For this review, take the finished solid that the model builds, in its own axes (mm). A direction names the side the tool comes from. Coordinates: 2 decimals unless noted, no trailing zeros. Order: outer loops, then holes, each group sorted by start corner. A loop starts at its lowest first (then second) coordinate and runs counter-clockwise, first axis right, second up. Notation, with made-up numbers: (37.5, 86) - (56.5, 86) arc R30 cw to (56.5, 123) - close; hole circle Ø8 at (89.5, 12). An arc over 180 degrees is marked (long way). One line per item, written item: value. Start each with the question number.
(1) Consider section A-A on z = 5. Write out the cut boundary in (x, y), then the cut area to 3 significant figures.
(2) Consider section D-D on y = 10. Write out the cut boundary in (x, z).
(3) Clearance check with flat-ended pins moving along their axes: pin 1 (0.7 mm diameter, centred on x = -0.5, z = 2, fed in from +Y); pin 2 (0.7 mm diameter, centred on x = 5.5, y = 2.5, fed in from -Z); pin 3 (5 mm diameter, centred on x = 2.54, y = 15.77, fed in from +Z). State where each tip first meets the part, or that it passes through.
(4) Mouldability with a two-part tool opening along Y and no side actions: class faces 1 (the flat face through (2.47, 12.15, -1.73)), 2 (the flat face through (2.5, 1, -1.28)), 3 (the flat face through (5.96, 0, 1)) as released by +Y, released by -Y, zero draft, split by the parting line, or undercut.
(5) Consider section B-B on x = 2.54. Write out the cut boundary in (y, z) (3 decimals).
(6) Consider section C-C on y = 15.77. Write out the cut boundary in (x, z) (3 decimals).
(7) To check wall thickness, follow line 1 along Y through (x, z) = (2.54, -4.35) (3 decimals); line 2 along Z through (x, y) = (6.5, 17); line 3 along Z through (x, y) = (5, 10.5). State the ranges of each line that lie inside material, in increasing order.
(8) For faces 4 (the cylindrical face through (2.5, -2.2, -1.1)), 5 (the flat face through (-0.88, 0, 1)), 6 (the flat face through (2.5, 1, -1.92)), 7 (the flat face through (3, 7, 0)), list the 3-axis set-ups (+Z, -Z, +X, -X, +Y, -Y) from which the entire face can be reached by the end or side of a thin tool; tool diameter is ignored.
```python
from build123d import *

# Parameters (mm, degrees)
SKETCH_5_W                      = 10.3
SKETCH_5_H                      = 4.8
EXTRUDE_1_DEPTH                 = 15.75
CUT_EXTRUDE_1_REACH             = 23.278
CUT_EXTRUDE_1_DIRECTION_2_REACH = 23.278
SKETCH_11_R                     = 1.865
CUT_EXTRUDE_2_DEPTH             = 4.8
SKETCH_3_W                      = 0.84
SKETCH_3_H                      = 0.64
SKETCH_4_W                      = 0.84
SKETCH_4_H                      = 0.64
SKETCH_3_3_W                    = 0.84
SKETCH_3_3_H                    = 0.64
EXTRUDE_2_DEPTH                 = 2.5
SKETCH_4_3_W                    = 0.84
SKETCH_4_3_H                    = 0.64
EXTRUDE_3_DEPTH                 = 2.5
SKETCH_12_W                     = 0.84
SKETCH_12_H                     = 0.64
EXTRUDE_4_DEPTH                 = 4
EXTRUDE_5_DEPTH                 = 0.46
EXTRUDE_6_DEPTH                 = 0.46
CUT_EXTRUDE_3_DEPTH             = 0.46
CUT_EXTRUDE_START               = -0.46
CUT_EXTRUDE_4_DEPTH             = 0.46
SKETCH_17_R                     = 0.172950306
CUT_EXTRUDE_5_DEPTH             = 2
SKETCH_18_W                     = 11.930877945
SKETCH_18_H                     = 3.370946467
CUT_EXTRUDE_6_DEPTH             = 2
EXTRUDE_7_DEPTH                 = 0.84


with BuildPart() as part:
    # Эскиз5 → Вытянуть1 (new body)
    with BuildSketch(Plane(origin=(0, 3.5, 0), x_dir=(-1, 0, 0), z_dir=(0, 1, 0))):
        with Locations((-2.54, -2.4)):
            Rectangle(SKETCH_5_W, SKETCH_5_H)
    extrude(amount=EXTRUDE_1_DEPTH)

    # Вырез-Вытянуть1: up to this face of the body (flat: up to its plane)
    cut_extrude_1_end = Plane(part.part.faces().sort_by_distance((-2.61, 11.375, -2.4))[0])
    # Эскиз10 → Вырез-Вытянуть1 (cut, up to the picked face)
    with BuildSketch(Plane(origin=(0, 0, 0), x_dir=(0, 0, -1), z_dir=(1, 0, 0)), mode=Mode.PRIVATE) as cut_extrude_1_sk1:
        Polygon((0, 19.25), (3.41, 19.25), (3.41, 12.78), (0, 11.5), align=None)
    cut_extrude_1_tool1 = split(extrude(cut_extrude_1_sk1.sketch, amount=-CUT_EXTRUDE_1_REACH, mode=Mode.PRIVATE), bisect_by=cut_extrude_1_end, keep=Keep.BOTH, mode=Mode.PRIVATE)
    add(cut_extrude_1_tool1.solids().sort_by(Axis((0, 15.685398, -1.653842), (-1, 0, 0)))[0], mode=Mode.SUBTRACT)

    # Вырез-Вытянуть1 direction 2: up to this face of the body (flat: up to its plane)
    cut_extrude_1_direction_2_end = Plane(part.part.faces().sort_by_distance((7.69, 11.375, -2.4))[0])
    # Эскиз10 → Вырез-Вытянуть1 direction 2 (cut, up to the picked face)
    with BuildSketch(Plane(origin=(0, 0, 0), x_dir=(0, 0, -1), z_dir=(1, 0, 0)), mode=Mode.PRIVATE) as cut_extrude_1_direction_2_sk1:
        Polygon((0, 19.25), (3.41, 19.25), (3.41, 12.78), (0, 11.5), align=None)
    cut_extrude_1_direction_2_tool1 = split(extrude(cut_extrude_1_direction_2_sk1.sketch, amount=CUT_EXTRUDE_1_DIRECTION_2_REACH, mode=Mode.PRIVATE), bisect_by=cut_extrude_1_direction_2_end, keep=Keep.BOTH, mode=Mode.PRIVATE)
    add(cut_extrude_1_direction_2_tool1.solids().sort_by(Axis((0, 15.685398, -1.653842), (1, 0, 0)))[0], mode=Mode.SUBTRACT)

    # Эскиз11 → Вырез-Вытянуть2 (cut)
    with BuildSketch(Plane.XY):
        with Locations((2.54, 15.77)):
            Circle(SKETCH_11_R)
    extrude(amount=-CUT_EXTRUDE_2_DEPTH, mode=Mode.SUBTRACT)

    # По траектории1: sweep along a path in Эскиз8
    with BuildLine(Plane(origin=(0, 0, 0), x_dir=(0, 0, -1), z_dir=(1, 0, 0))) as sweep_1_path:
        Line((0, 0), (0.6, 0))
        ThreePointArc((0.6, 0), (1.307106781, 0.292893219), (1.6, 1))
        Line((1.6, 1), (1.6, 3.5))
    # Эскиз3 → По траектории1 (sweep)
    with BuildSketch(Plane.XY):
        Rectangle(SKETCH_3_W, SKETCH_3_H)
        with Locations((5.08, 0)):
            Rectangle(SKETCH_3_W, SKETCH_3_H)
    sweep(path=sweep_1_path.line)

    # По траектории2: sweep along a path in Эскиз9
    with BuildLine(Plane(origin=(0, 0, 0), x_dir=(0, 0, -1), z_dir=(1, 0, 0))) as sweep_2_path:
        Line((0, -2.54), (0.6, -2.54))
        ThreePointArc((0.6, -2.54), (1.307106781, -2.247106781), (1.6, -1.54))
        Line((1.6, -1.54), (1.6, 4.77))
    # Эскиз4 → По траектории2 (sweep)
    with BuildSketch(Plane.XY):
        with Locations((2.54, -2.54)):
            Rectangle(SKETCH_4_W, SKETCH_4_H)
    sweep(path=sweep_2_path.line)

    # Эскиз3<3> → Вытянуть2 (add)
    with BuildSketch(Plane.XY):
        Rectangle(SKETCH_3_3_W, SKETCH_3_3_H)
        with Locations((5.08, 0)):
            Rectangle(SKETCH_3_3_W, SKETCH_3_3_H)
    extrude(amount=EXTRUDE_2_DEPTH)

    # Эскиз4<3> → Вытянуть3 (add)
    with BuildSketch(Plane.XY):
        with Locations((2.54, -2.54)):
            Rectangle(SKETCH_4_3_W, SKETCH_4_3_H)
    extrude(amount=EXTRUDE_3_DEPTH)

    # Эскиз12 → Вытянуть4 (add)
    with BuildSketch(Plane.XY.offset(2.5)):
        Rectangle(SKETCH_12_W, SKETCH_12_H)
        with Locations((5.08, 0)):
            Rectangle(SKETCH_12_W, SKETCH_12_H)
        with Locations((2.54, -2.54)):
            Rectangle(SKETCH_12_W, SKETCH_12_H)
    extrude(amount=EXTRUDE_4_DEPTH)

    # Эскиз13 → Вытянуть5 (add)
    with BuildSketch(Plane.ZY.offset(0.42)):
        with BuildLine():
            Line((-0.6, -0.32), (6.5, -0.32))
            Line((6.5, -0.32), (6.5, 0.32))
            Line((6.5, 0.32), (-0.6, 0.32))
            ThreePointArc((-0.6, 0.32), (-1.080832611, 0.519167389), (-1.28, 1))
            Line((-1.28, 1), (-1.28, 3.5))
            Line((-1.28, 3.5), (-1.92, 3.5))
            Line((-1.92, 3.5), (-1.92, 1))
            ThreePointArc((-1.92, 1), (-1.533380951, 0.066619049), (-0.6, -0.32))
        make_face()
    extrude(amount=EXTRUDE_5_DEPTH)

    # Эскиз14 → Вытянуть6 (add)
    with BuildSketch(Plane(origin=(5.5, 0, 0), x_dir=(0, 0, -1), z_dir=(1, 0, 0))):
        with BuildLine():
            Line((0.6, 0.32), (-6.5, 0.32))
            Line((-6.5, 0.32), (-6.5, -0.32))
            Line((-6.5, -0.32), (0.6, -0.32))
            ThreePointArc((0.6, -0.32), (1.533380951, 0.066619049), (1.92, 1))
            Line((1.92, 1), (1.92, 3.5))
            Line((1.92, 3.5), (1.28, 3.5))
            Line((1.28, 3.5), (1.28, 1))
            ThreePointArc((1.28, 1), (1.080832611, 0.519167389), (0.6, 0.32))
        make_face()
    extrude(amount=EXTRUDE_6_DEPTH)

    # Эскиз15 → Вырез-Вытянуть3 (cut)
    with BuildSketch(Plane.ZY.offset(-4.66)):
        with BuildLine():
            Line((-0.6, -0.32), (6.5, -0.32))
            Line((6.5, -0.32), (6.5, 0.32))
            Line((6.5, 0.32), (-0.6, 0.32))
            ThreePointArc((-0.6, 0.32), (-1.080832611, 0.519167389), (-1.28, 1))
            Line((-1.28, 1), (-1.28, 3.5))
            Line((-1.28, 3.5), (-1.92, 3.5))
            Line((-1.92, 3.5), (-1.92, 1))
            ThreePointArc((-1.92, 1), (-1.533380951, 0.066619049), (-0.6, -0.32))
        make_face()
    extrude(amount=-CUT_EXTRUDE_3_DEPTH, mode=Mode.SUBTRACT)

    # Эскиз16 → Вырез-Вытянуть4 (cut)
    with BuildSketch(Plane(origin=(0.42, 0, 0), x_dir=(0, 0, -1), z_dir=(1, 0, 0)).offset(CUT_EXTRUDE_START)):
        with BuildLine():
            Line((0.6, 0.32), (-6.5, 0.32))
            Line((-6.5, 0.32), (-6.5, -0.32))
            Line((-6.5, -0.32), (0.6, -0.32))
            ThreePointArc((0.6, -0.32), (1.533380951, 0.066619049), (1.92, 1))
            Line((1.92, 1), (1.92, 3.5))
            Line((1.92, 3.5), (1.28, 3.5))
            Line((1.28, 3.5), (1.28, 1))
            ThreePointArc((1.28, 1), (1.080832611, 0.519167389), (0.6, 0.32))
        make_face()
    extrude(amount=CUT_EXTRUDE_4_DEPTH, mode=Mode.SUBTRACT)

    # Эскиз17 → Вырез-Вытянуть5 (cut)
    with BuildSketch(Plane.XY.offset(6.5)):
        with Locations((-0.46, 0)):
            Circle(SKETCH_17_R)
    extrude(amount=-CUT_EXTRUDE_5_DEPTH, mode=Mode.SUBTRACT)

    # Эскиз18 → Вырез-Вытянуть6 (cut)
    with BuildSketch(Plane.ZY.offset(-2.12)):
        with Locations((2.005211992, -3.225473234)):
            Rectangle(SKETCH_18_W, SKETCH_18_H)
    extrude(amount=-CUT_EXTRUDE_6_DEPTH, mode=Mode.SUBTRACT)

    # Эскиз19 → Вытянуть7 (add)
    with BuildSketch(Plane.ZY.offset(-2.12)):
        with BuildLine():
            Line((-0.6, -3.32), (6.5, -3.32))
            Line((6.5, -3.32), (6.5, -2.68))
            Line((6.5, -2.68), (-0.6, -2.68))
            ThreePointArc((-0.6, -2.68), (-1.097088212, -2.20370174), (-1.28, -1.54))
            Line((-1.28, -1.54), (-1.92, -1.54))
            ThreePointArc((-1.92, -1.54), (-1.553991604, -2.648016245), (-0.6, -3.32))
        make_face()
    extrude(amount=-EXTRUDE_7_DEPTH)


solid = part.part
```
Geometry check:
1. outline: (-0.88, -0.32) - (-0.04, -0.32) - (-0.04, 0.32) - (-0.88, 0.32) - close; (2.12, -3.32) - (2.96, -3.32) - (2.96, -2.68) - (2.12, -2.68) - close; (5.12, -0.32) - (5.96, -0.32) - (5.96, 0.32) - (5.12, 0.32) - close; hole circle Ø0.35 at (-0.46, 0)
1. area: 1.52 mm^2
2. outline: (-2.61, -4.8) - (7.69, -4.8) - (7.69, 0) - (-2.61, 0) - close
3. pin 1: stops at y = 0.32
3. pin 2: stops at z = -1.92
3. pin 3: stops at z = -3.41
4. face 1: released by +Y
4. face 2: undercut
4. face 3: zero draft
5. outline: (-3.32, -0.6) arc R1.86 ccw to (-1.54, -1.92) - (3.5, -1.92) - (3.5, -4.8) - (13.905, -4.8) - (13.905, -3.41) - (12.78, -3.41) - (11.5, 0) - (3.5, 0) - (3.5, -1.28) - (-1.54, -1.28) arc R1.296 cw to (-2.68, -0.6) - (-2.68, 6.5) - (-3.32, 6.5) - close; (17.635, -4.8) - (19.25, -4.8) - (19.25, -3.41) - (17.635, -3.41) - close
6. outline: (-2.61, -4.8) - (0.675, -4.8) - (0.675, -3.41) - (-2.61, -3.41) - close; (4.405, -4.8) - (7.69, -4.8) - (7.69, -3.41) - (4.405, -3.41) - close
7. line 1: y = 3.5 to 13.905, 17.635 to 19.25
7. line 2: z = -4.8 to -3.41
7. line 3: z = -4.8 to 0
8. face 4: +Z, +X, -X
8. face 5: +Z, -Z, -X, -Y
8. face 6: -Z, +X, -X, -Y
8. face 7: +Z, +X, -X, +Y
